from build123d import *

# Parameters (mm, degrees)
F1_DEPTH = 25.4


with BuildPart() as f1:
    # F0 (on Front) → F1 (new body)
    with BuildSketch(Plane.XZ):
        with BuildLine():
            Line((-114.3, 0), (139.7, 0))
            ThreePointArc((139.7, 0), (-139.116658, 12.753253), (137.371504, -25.4))
            Line((137.371504, -25.4), (111.442048, -25.4))
            ThreePointArc((111.442048, -25.4), (-12.78014, -113.583265), (-114.3, 0))
        make_face()
        with BuildLine():
            ThreePointArc((-111.442048, 25.4), (0, 114.3), (111.442048, 25.4))
            Line((111.442048, 25.4), (-111.442048, 25.4))
        make_face(mode=Mode.SUBTRACT)
    extrude(amount=F1_DEPTH)


solid = f1.part
Verification items for the finished model (mm, model axes). A direction names the side the tool comes from. Give positions to 0.01 mm unless a question says otherwise; leave off trailing zeros. Loops run counter-clockwise (first coordinate to the right, second up) from the corner with the lowest first, then second, coordinate; pieces in that order, holes last. Notation, with made-up numbers: (49, 13.25) - (53, 13.25) arc R17 ccw to (53, 36.25) - close; hole circle Ø8 at (-6.75, 42). An arc over 180 degrees is marked (long way). Write item = value, one per line. Start each with the question number.
Q1. Cross-section at D-D, the plane x = -67. Enter the section's corners in (y, z).
Q2. Cross-section at C-C, the plane y = -15.75. Enter the section's corners in (x, z).
Q3. Thickness scan on line 1 (Z direction, x = -70, y = -9.5); line 2 (Z direction, x = -78.5, y = -4.5); line 3 (X direction, y = -12, z = 79). Record the ranges inside material, lowest first.
Q4. Mould release check, pull along Z, two halves, no side actions. Record for faces 4 (the face through (-1, -25.4, 11)), 5 (the face through (-138.445, -12.522, 18.68)), 6 (the face through (-2.15, -12.52, 114.28)): released by +Z, released by -Z, zero draft, split by the parting line, or undercut.
Q5. Cross-section at A-A, the plane x = 0. Enter the section's corners in (y, z).
Q6. Depth check by flat-ended pin: P1, Ø6, axis at x = 60.5, y = -11.5, coming from the +Z side; P2, Ø3, axis at y = -6.5, z = 67.5, coming from the +X side; P3, Ø7.5, axis at x = 122, y = -16.5, coming from the +Z side. Enter the tip coordinate at first touch or a pass-through.
Q7. Tool access check on faces 1 (the face through (-1, 0, 11)), 2 (the face through (-10.46, -12.52, -113.82)), 3 (the face through (11, -13, 0)). Record the directions out of +Z, -Z, +X, -X, +Y, -Y that give a thin tool (end or side, any length) a straight path to the whole face; none if there is none.
Q8. Cross-section at B-B, the plane z = 59. Enter the section's corners in (x, y), and give its area (3 significant figures).
Answer key:
q1.outline = (-25.4, -122.59) - (0, -122.59) - (0, -92.6) - (-25.4, -92.6) - close; (-25.4, 0) - (0, 0) - (0, 25.4) - (-25.4, 25.4) - close; (-25.4, 92.6) - (0, 92.6) - (0, 122.59) - (-25.4, 122.59) - close
q2.outline = (-114.3, 0) - (139.7, 0) arc R139.7 ccw (long way) to (137.37, -25.4) - (111.44, -25.4) arc R114.3 cw to start; hole (-111.44, 25.4) - (111.44, 25.4) arc R114.3 ccw to start
q3.line_1 = -120.9 to -90.36, 0 to 25.4, 90.36 to 120.9
q3.line_2 = -115.56 to -83.08, 0 to 25.4, 83.08 to 115.56
q3.line_3 = -115.22 to -82.6, 82.6 to 115.22
q4.face_4 = zero draft
q4.face_5 = split by the parting line
q4.face_6 = undercut
q5.outline = (-25.4, -139.7) - (0, -139.7) - (0, -114.3) - (-25.4, -114.3) - close; (-25.4, 0) - (0, 0) - (0, 25.4) - (-25.4, 25.4) - close; (-25.4, 114.3) - (0, 114.3) - (0, 139.7) - (-25.4, 139.7) - close
q6.P1 = 127.32
q6.P2 = 123.13
q6.P3 = 74.38
q7.face_1 = +Z, -Z, +X, -X, +Y
q7.face_2 = +Y, -Y
q7.face_3 = +X, +Y, -Y
q8.outline = (-126.63, -25.4) - (-97.9, -25.4) - (-97.9, 0) - (-126.63, 0) - close; (97.9, -25.4) - (126.63, -25.4) - (126.63, 0) - (97.9, 0) - close
q8.area = 1,460 mm^2
